Answer from the drawing. Dimensions are ordinates in mm from the lowest x, y and z of the part. Round coordinates to 2 decimals unless told otherwise and drop trailing zeros. Loops run counter-clockwise (first coordinate to the right, second up) from the corner with the lowest first, then second, coordinate; pieces in that order, holes last.
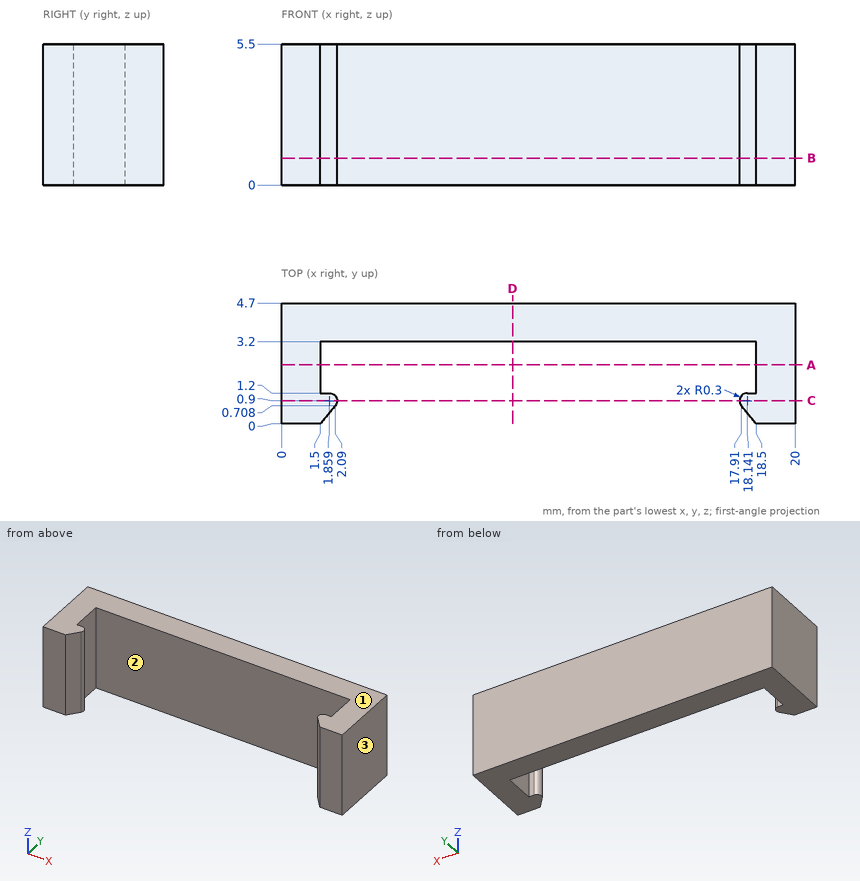
1. Find section D-D (x = 9). Write down the section's boundary in (y, z).
Answer key:
outline: (3.2, 0) - (4.7, 0) - (4.7, 5.5) - (3.2, 5.5) - close
2. Determine the mould class of the marked faces 1, 2 and 3 for opening direction X: +X half, -X half, draft (parallel to the pull), parting line (faces both ways), or undercut.
Answer key:
face 1: draft
face 2: undercut
face 3: +X half
3. Find section B-B (z = 1.05). Write down the section's boundary in (x, y).
Answer key:
outline: (0, 0) - (1.5, 0) - (2.09, 0.71) arc R0.3 ccw to (1.86, 1.2) - (1.5, 1.2) - (1.5, 3.2) - (18.5, 3.2) - (18.5, 1.2) - (18.14, 1.2) arc R0.3 ccw to (17.91, 0.71) - (18.5, 0) - (20, 0) - (20, 4.7) - (0, 4.7) - close
4. Given pin 1 (3 mm diameter, centred on x = 9, z = 2, fed in from -Y); pin 2 (3 mm diameter, centred on x = 17.5, z = 3.5, fed in from -Y), each flat-ended and moving along its own axis, determine where each tip first touches the part or whether it passes through.
Answer key:
pin 1: stops at y = 3.2
pin 2: stops at y = 0
5. Find section C-C (y = 0.9). Write down the section's boundary in (x, z).
Answer key:
outline: (0, 0) - (2.16, 0) - (2.16, 5.5) - (0, 5.5) - close; (17.84, 0) - (20, 0) - (20, 5.5) - (17.84, 5.5) - close
6. Consider probe 1 along X at (y, z) = (2.4, 0.5); probe 2 along Y at (x, z) = (11.25, 3.6); probe 3 along Y at (x, z) = (2, 1.5) (1 decimal). Determine where each line is inside the solid, lowest interval first.
Answer key:
probe 1: x = 0 to 1.5, 18.5 to 20
probe 2: y = 3.2 to 4.7
probe 3: y = 0.6 to 1.2, 3.2 to 4.7
7. Find section A-A (y = 2.3). Write down the section's boundary in (x, z).
Answer key:
outline: (0, 0) - (1.5, 0) - (1.5, 5.5) - (0, 5.5) - close; (18.5, 0) - (20, 0) - (20, 5.5) - (18.5, 5.5) - close
